Autodesk Inventor part; units mm, degrees
ref_plane "YZ Plane" through (0, 0, 0) normal (1, 0, 0) x (0, 1, 0)
ref_plane "XZ Plane" through (0, 0, 0) normal (0, 1, 0) x (-1, 0, 0)
ref_plane "XY Plane" through (0, 0, 0) normal (0, 0, 1) x (1, 0, 0)
sketch "Sketch1" plane through (0, 0, 0) normal (0, 1, 0) x (-1, 0, 0)
  line L0 (-50, 50) -> (50, 50)
  line L1 (50, 50) -> (50, -50)
  line L2 (50, -50) -> (-50, -50)
  line L3 (-50, -50) -> (-50, 50)
  line L4 (-50, 50) -> (50, -50) construction
  line L5 (50, 50) -> (-50, -50) construction
  circle A0 centre (0, 0) radius 30
  line L6 (-35.5, 35.5) -> (35.5, 35.5) construction
  line L7 (35.5, 35.5) -> (35.5, -35.5) construction
  line L8 (35.5, -35.5) -> (-35.5, -35.5) construction
  line L9 (-35.5, -35.5) -> (-35.5, 35.5) construction
  line L10 (-35.5, 35.5) -> (35.5, -35.5) construction
  line L11 (35.5, 35.5) -> (-35.5, -35.5) construction
  dimension "d0" = 100
  dimension "d1" = 60
  dimension "d2" = 71
  dimension "d13" = 100.4092
extrude "Extrusion1" add sketch "Sketch1" against normal blind 15
hole "Hole1" at (-35.5, 0, -35.5) at (35.5, 0, -35.5) at (35.5, 0, 35.5) at (-35.5, 0, 35.5) direction (0, -1, 0) diameter 7 end through all counterbore diameter 12 counterbore depth 6
fillet "Fillet1" radius 12 4 edges at (-50, -7.5, -50) (50, -7.5, -50) (50, -7.5, 50) (-50, -7.5, 50)
properties part number "MP1-001" material "Wood (Birch)"
The model under review builds one solid part; all positions refer to its coordinate system, in mm. A direction names the side the tool comes from. Give positions to 0.01 mm unless a question says otherwise; leave off trailing zeros. Loops run counter-clockwise (first coordinate to the right, second up) from the corner with the lowest first, then second, coordinate; pieces in that order, holes last. Notation, with made-up numbers: (1.5, 5.5) -> (54.5, 5.5) arc R21 ccw to (54.5, 31.5) -> close; hole circle Ø6 at (51.5, 64.5). An arc over 180 degrees is marked (long way). Answer as a JSON object with one key per item and string values. Group by question number.
Q1. Take a section at A-A (y = -10.25). Write out the cut boundary in (x, z), plus the area to 4 significant figures.
Q2. Insertion check: pin 1 (9.5 mm diameter, centred on x = -34, z = -32.5, fed in from +Y); pin 2 (6 mm diameter, centred on x = 36, z = 35, fed in from +Y). Each pin has a flat end and moves straight along its axis. Give the tip position at first contact, or say it passes through.
Q3. Tool access review of faces 1 (the cylindrical face through (39.15, -3.04, 30.74)), 2 (the flat face through (-1, -7, -50)): name each direction out of +Z, -Z, +X, -X, +Y, -Y from which nothing blocks a thin tool from reaching the whole face with its end or side.
Q4. Wall thickness on line 1 along X through (y, z) = (-4.25, 35.5); line 2 along X through (y, z) = (-13, 35.5): over which ranges is each line inside the solid? List them lowest first.
Q5. Draft analysis for pull direction Z (two halves, no side actions). For faces 3 (the cylindrical face through (-46.58, -7.6, -46.39)), 4 (the cylindrical face through (-31.85, -3.04, -40.26)), 5 (the flat face through (38.1, -6, 38.1)), 6 (the cylindrical face through (-46.39, -7.6, 46.58)), state which applies: pulls with the +Z half, pulls with the -Z half, needs draft (parallel to the pull), parting line crosses it, or undercut.
Q6. Take a section at C-C (x = 35.5). Write out the cut boundary in (y, z), plus the area to 3 significant figures.
Q7. Take a section at B-B (z = -24). Write out the cut boundary in (x, y).
Q8. Take a section at D-D (x = 0). Write out the cut boundary in (y, z).
Answer below:
{
 "1": {"outline": "(-50, -38) arc R12 ccw to (-38, -50) -> (38, -50) arc R12 ccw to (50, -38) -> (50, 38) arc R12 ccw to (38, 50) -> (-38, 50) arc R12 ccw to (-50, 38) -> close; hole circle Ø7 at (-35.5, -35.5); hole circle Ø7 at (-35.5, 35.5); hole circle Ø60 at (0, 0); hole circle Ø7 at (35.5, -35.5); hole circle Ø7 at (35.5, 35.5)", "area": "6,895 mm2"},
 "2": {"pin 1": "stops at y = 0", "pin 2": "stops at y = -6"},
 "3": {"face 1": "+Y", "face 2": "-Z, +X, -X, +Y, -Y"},
 "4": {"line 1": "x = -50 to -41.5, -29.5 to 29.5, 41.5 to 50", "line 2": "x = -50 to -39, -32 to 32, 39 to 50"},
 "5": {"face 3": "pulls with the -Z half", "face 4": "undercut", "face 5": "undercut", "face 6": "pulls with the +Z half"},
 "6": {"outline": "(-15, -50) -> (0, -50) -> (0, -41.5) -> (-6, -41.5) -> (-6, -39) -> (-15, -39) -> close; (-15, -32) -> (-6, -32) -> (-6, -29.5) -> (0, -29.5) -> (0, 29.5) -> (-6, 29.5) -> (-6, 32) -> (-15, 32) -> close; (-15, 39) -> (-6, 39) -> (-6, 41.5) -> (0, 41.5) -> (0, 50) -> (-15, 50) -> close", "area": "1,230 mm2"},
 "7": {"outline": "(-50, -15) -> (-18, -15) -> (-18, 0) -> (-50, 0) -> close; (18, -15) -> (50, -15) -> (50, 0) -> (18, 0) -> close"},
 "8": {"outline": "(-15, -50) -> (0, -50) -> (0, -30) -> (-15, -30) -> close; (-15, 30) -> (0, 30) -> (0, 50) -> (-15, 50) -> close"}
}
